```python
from build123d import *

# Parameters (mm, degrees)
EXTRUDE_1_DEPTH          = 10
SKETCH_2_R               = 335.5
EXTRUDE_2_DEPTH          = 196
EXTRUDE_3_DEPTH          = 154.8
SHELL_START              = 10
SHELL_1_OUTLINE_R        = 330.5
SHELL_1_DEPTH            = 191
SHELL_1_2_DEPTH          = 149.8
CUT_EXTRUDE_4_DEPTH      = 632.790169442
EXTRUDE_4_DEPTH          = 61.8
EXTRUDE_4_DEPTH_BACK     = 128.6
SKETCH_6_R               = 80
SKETCH_9_R               = 75
CUT_EXTRUDE_5_DEPTH      = 185.4
SKETCH_10_R              = 10
CUT_EXTRUDE_6_DEPTH      = 654.608184009
PATTERN_CIRCULAR_1_COUNT = 4
RIB_START                = -5
RIB_1_DEPTH              = 10
PATTERN_CIRCULAR_3_COUNT = 6
RIB_2_REACH              = 659.617
SKETCH_12_WALL_W         = 1579.41836799
SKETCH_12_WALL_H         = 10
SKETCH_13_R              = 48
CUT_EXTRUDE_7_DEPTH      = 658.616649883
FILLET_1_R               = 10


# Read off the part's stored shape, not the designer's step: 抽壳1, 筋1
with BuildPart() as part:
    # 草图1 → 凸台-拉伸1 (new body)
    with BuildSketch(Plane.XY):
        with BuildLine():
            ThreePointArc((403.953420148, -194.523409518), (415.106395354, -169.423738113), (424.701552978, -143.688250731))
            Line((424.701552978, -143.688250731), (423.18702464, 148.0893807))
            ThreePointArc((423.18702464, 148.0893807), (413.325221182, 173.723872955), (401.91228456, 198.706411622))
            Line((401.91228456, 198.706411622), (194.523409518, 403.953420148))
            ThreePointArc((194.523409518, 403.953420148), (169.423738113, 415.106395354), (143.688250731, 424.701552978))
            Line((143.688250731, 424.701552978), (-148.0893807, 423.18702464))
            ThreePointArc((-148.0893807, 423.18702464), (-173.723872955, 413.325221182), (-198.706411622, 401.91228456))
            Line((-198.706411622, 401.91228456), (-403.953420148, 194.523409518))
            ThreePointArc((-403.953420148, 194.523409518), (-415.106395354, 169.423738113), (-424.701552978, 143.688250731))
            Line((-424.701552978, 143.688250731), (-423.18702464, -148.0893807))
            ThreePointArc((-423.18702464, -148.0893807), (-413.325221182, -173.723872955), (-401.91228456, -198.706411622))
            Line((-401.91228456, -198.706411622), (-194.523409518, -403.953420148))
            ThreePointArc((-194.523409518, -403.953420148), (-169.423738113, -415.106395354), (-143.688250731, -424.701552978))
            Line((-143.688250731, -424.701552978), (148.0893807, -423.18702464))
            ThreePointArc((148.0893807, -423.18702464), (173.723872955, -413.325221182), (198.706411622, -401.91228456))
            Line((198.706411622, -401.91228456), (403.953420148, -194.523409518))
        make_face()
    extrude(amount=EXTRUDE_1_DEPTH)

    # 草图4 → 切除-拉伸4 (cut, through all)
    with BuildSketch(Plane(origin=(0, 0, 10), x_dir=(-1, 0, 0), z_dir=(0, 0, -1))):
        with BuildLine():
            Line((-295.51015211, -148), (-361, -148))
            Line((-361, -148), (-361, 148))
            Line((-361, 148), (-295.51015211, 148))
            ThreePointArc((-295.51015211, 148), (330.5, 0), (-295.51015211, -148))
        make_face()
    extrude(amount=CUT_EXTRUDE_4_DEPTH, mode=Mode.SUBTRACT)


with BuildPart() as body_2:
    # 草图2 → 凸台-拉伸2 (new body)
    with BuildSketch(Plane.XY.offset(10)):
        Circle(SKETCH_2_R)
    extrude(amount=EXTRUDE_2_DEPTH)


with BuildPart() as body_3:
    # 草图3 → 凸台-拉伸3 (new body)
    with BuildSketch(Plane.XY.offset(10)):
        with BuildLine():
            Line((366, -153), (366, 153))
            Line((366, 153), (298.582065771, 153))
            ThreePointArc((298.582065771, 153), (335.5, 0), (298.582065771, -153))
            Line((298.582065771, -153), (366, -153))
        make_face()
    extrude(amount=EXTRUDE_3_DEPTH)


with BuildPart() as body_2_1:
    add(body_2.part)

    # Combine 1: union body 3
    add(body_3.part)

    # 抽壳1 outline → 抽壳1 (cut)
    with BuildSketch(Plane.XY.offset(SHELL_START)):
        Circle(SHELL_1_OUTLINE_R)
    extrude(amount=SHELL_1_DEPTH, mode=Mode.SUBTRACT)

    # Shell 1 2 outline → Shell 1 2 (cut)
    with BuildSketch(Plane.XY.offset(SHELL_START)):
        with BuildLine():
            ThreePointArc((295.51015211, 148), (330.5, 0), (295.51015211, -148))
            Line((295.51015211, -148), (361, -148))
            Line((361, -148), (361, 148))
            Line((361, 148), (295.51015211, 148))
        make_face()
    extrude(amount=SHELL_1_2_DEPTH, mode=Mode.SUBTRACT)

    # Combine 2: union part
    add(part.part)

    # 草图6 → 凸台-拉伸4 (add, two sides: drawn at the far end of the back side and taken through both)
    with BuildSketch(Plane.XY.offset(206).offset(-EXTRUDE_4_DEPTH_BACK)):
        Circle(SKETCH_6_R)
    extrude(amount=EXTRUDE_4_DEPTH + EXTRUDE_4_DEPTH_BACK)

    # 草图9 → 切除-拉伸5 (cut)
    with BuildSketch(Plane(origin=(0, 0, 77.4), x_dir=(-1, 0, 0), z_dir=(0, 0, -1))):
        Circle(SKETCH_9_R)
    extrude(amount=-CUT_EXTRUDE_5_DEPTH, mode=Mode.SUBTRACT)

    # 草图10 → 切除-拉伸6 (cut, through all)
    with BuildSketch(Plane.XY.offset(10)):
        with Locations((-232.660524103, 307.498096619)):
            Circle(SKETCH_10_R)
        with Locations((-309.896801034, 229.455816246)):
            Circle(SKETCH_10_R)
    cut_extrude_6 = extrude(amount=-CUT_EXTRUDE_6_DEPTH, mode=Mode.SUBTRACT)

    # 阵列(圆周)1: 切除-拉伸6 ×4 about axis
    pattern_circular_1_axis = Axis((0, 0, 0), (0, 0, 1))
    for i in range(1, PATTERN_CIRCULAR_1_COUNT):
        add(cut_extrude_6.rotate(pattern_circular_1_axis, i * 360 / PATTERN_CIRCULAR_1_COUNT), mode=Mode.SUBTRACT)

    # 筋1 outline → 筋1 (add)
    with BuildSketch(Plane(origin=(0, 0, 0), x_dir=(1, 0, 0), z_dir=(0, 1, 0)).offset(RIB_START)):
        Polygon((-79.843597113, -82.38631652), (-330.5, -104.315910213), (-332, -104.447143208), (-332, -201), (-78, -201), (-78, -82.225022673), align=None)
    rib_1 = extrude(amount=RIB_1_DEPTH)

    # 阵列(圆周)3: 筋1 ×6 about axis, 1 skipped
    pattern_circular_3_axis = Axis((0, 0, 0), (0, 0, 1))
    add([rib_1.rotate(pattern_circular_3_axis, i * 360 / PATTERN_CIRCULAR_3_COUNT) for i in range(1, PATTERN_CIRCULAR_3_COUNT) if i not in (3,)])

    # 草图12 wall → 筋2 (add, up to next)
    with BuildSketch(Plane(origin=(205.25, 0, 121.1), x_dir=(0.955431984347, 0, 0.295211319714), z_dir=(0.295211319714, 0, -0.955431984347)), mode=Mode.PRIVATE) as rib_2_sk1:
        Rectangle(SKETCH_12_WALL_W, SKETCH_12_WALL_H)
    rib_2_tool1 = extrude(rib_2_sk1.sketch, amount=-RIB_2_REACH, mode=Mode.PRIVATE) - body_2_1.part
    add(rib_2_tool1.solids().sort_by_distance((205.25, 0, 121.1))[0])

    # 草图13 → 切除-拉伸7 (cut, through all)
    with BuildSketch(Plane.XY.offset(267.8)):
        Circle(SKETCH_13_R)
    extrude(amount=-CUT_EXTRUDE_7_DEPTH, mode=Mode.SUBTRACT)

    # 圆角1
    fillet_1_edges = [body_2_1.edges().sort_by_distance(p)[0] for p in [
        (-335.5, 0, 206),
        (332.291032885, 153, 10),
        (366, 153, 87.4),
        (298.582065771, 153, 87.4),
        (332.291032885, -153, 10),
        (298.582065771, -153, 87.4),
        (366, 0, 10),
        (366, -153, 87.4),
        (326.139949306, 78.695511098, 164.8),
        (366, 0, 164.8),
    ]]
    fillet(fillet_1_edges, radius=FILLET_1_R)


solid = body_2_1.part
```
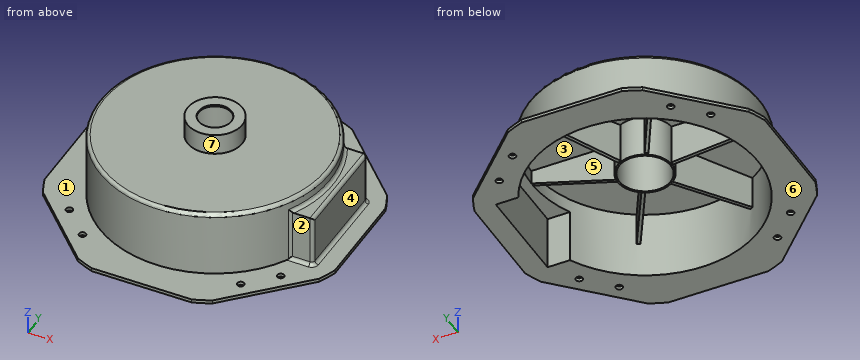
Source: CAD feature listing. Evaluate the final solid. Frame: model axes, mm. Face numbers are marked on the shaded views. A direction names the side the tool comes from. Coordinates: 2 decimals unless noted, no trailing zeros. Write each loop counter-clockwise with the first axis right and the second up, starting at its lowest first coordinate (ties: lowest second). Pieces come first, ordered by that corner, then holes. Notation, with made-up numbers: (0, 42) -> (56, 42) arc R18 ccw to (56, 65) -> close; hole circle Ø6 at (1, 58). An arc over 180 degrees is marked (long way). Return JSON: item names as keys, results as strings. Group by question number.
1) Set-up query: the marked faces 1, 2, 3 and 4. Return all of +Z, -Z, +X, -X, +Y, -Y with unobstructed straight access to the full face (end or side cutting, diameter ignored); none if empty.
2) Contact query for flat-ended pins moving along their axis: P1, Ø2, axis at y = 255.5, z = 173.5, coming from the -X side; P2, Ø8, axis at y = -57, z = 178.5, coming from the -X side; P3, Ø4, axis at y = -258, z = 59, coming from the +X side. Output: stop coordinate, or through.
3) Mould query, pull axis Y, two halves, no side actions, for the marked faces 5, 6 and 7. Classes: +Y half, -Y half, draft (parallel to the pull), parting line (faces both ways), or undercut.
4) Section query C-C, the plane z = 224. Return loops of the section in (x, y), plus the area to 3 significant figures.
5) Ray query, line 1 along Y through (x, z) = (0, 189.5); line 2 along Y through (x, z) = (-106.5, 107.5); line 3 along Y through (x, z) = (0, 265.25). Return the intervals inside material, ascending.
6) Section query A-A, the plane z = 32. Return loops of the section in (x, y).
From the geometry:
{
 "1": {"face 1": "+Z", "face 2": "+Z, +X, -Y", "face 3": "-Z", "face 4": "+Z, +X, +Y, -Y"},
 "2": {"P1": "x = -218.61", "P2": "x = -331.29", "P3": "x = 216.85"},
 "3": {"face 5": "undercut", "face 6": "draft", "face 7": "parting line"},
 "4": {"outline": "circle Ø160 at (0, 0); hole circle Ø150 at (0, 0)", "area": "2,430 mm²"},
 "5": {"line 1": "-335.5 to -330.5, -80 to -75, 75 to 80, 330.5 to 335.5", "line 2": "-318.15 to -312.87, -194.46 to -174.46, -5 to 5, 174.46 to 194.46, 312.87 to 318.15", "line 3": "-80 to -48, 48 to 80"},
 "6": {"outline": "(295.82, -158.28) arc R10 cw to (304.63, -153) -> (356, -153) arc R10 ccw to (366, -143) -> (366, 143) arc R10 ccw to (356, 153) -> (304.63, 153) arc R10 cw to (295.82, 158.28) arc R335.5 ccw (long way) to start; hole (295.51, -148) -> (361, -148) -> (361, 148) -> (295.51, 148) arc R330.5 ccw (long way) to start"}
}
